from build123d import *

# Parameters (mm, degrees)
F0_W      = 111.801914
F0_H      = 111.801914
F1_DEPTH  = 57.15
F2_W      = 72.47591
F2_H      = 72.47591
F3_DEPTH  = 71.12
F4_W      = 21.19565
F4_H      = 21.19565
F5_DEPTH  = 76.2
F6_R      = 16.556677
F7_W      = 7.638184
F7_H      = 15.41857
F8_DEPTH  = 25.4
F8_FACE_W = 7.638184
F8_FACE_H = 15.41857
F9_DEPTH  = 27.432
F10_W     = 78.688562
F10_H     = 9.165822
F11_DEPTH = 8.89
F12_W     = 8.714252
F12_H     = 81.186646
F13_DEPTH = 8.636
F14_W     = 78.688562
F14_H     = 8.29689
F15_DEPTH = 15.748
F16_W     = 8.432022
F16_H     = 81.186646
F17_DEPTH = 12.446
F18_R     = 18.732784
F19_DEPTH = 1.778


with BuildPart() as f1:
    # F0 (on Top) → F1 (new body, symmetric)
    with BuildSketch(Plane.XY):
        Rectangle(F0_W, F0_H)
    extrude(amount=F1_DEPTH, both=True)

    # F2 (on face) → F3 (join)
    with BuildSketch(Plane.XZ.offset(55.900957)):
        Rectangle(F2_W, F2_H)
    extrude(amount=F3_DEPTH)

    # F4 (on face) → F5 (join)
    with BuildSketch(Plane.XZ.offset(127.020957)):
        Rectangle(F4_W, F4_H)
    extrude(amount=F5_DEPTH)

    # F6
    f6_edges = [f1.edges().sort_by_distance(p)[0] for p in [
        (-55.900957, 0, 57.15),
        (-55.900957, 0, -57.15),
        (55.900957, 0, -57.15),
        (55.900957, 0, 57.15),
        (36.237955, -127.020957, 0),
        (0, -127.020957, -36.237955),
        (-36.237955, -127.020957, 0),
        (0, -127.020957, 36.237955),
        (-36.237955, -91.460957, -36.237955),
        (36.237955, -91.460957, -36.237955),
        (36.237955, -91.460957, 36.237955),
        (-36.237955, -91.460957, 36.237955),
    ]]
    fillet(f6_edges, radius=F6_R)

    # F7 (on face) → F8 (join)
    with BuildSketch(Plane.XY.offset(57.15)):
        with Locations((-30.17084, 48.191672)):
            Rectangle(F7_W, F7_H)
    extrude(amount=F8_DEPTH)

    # F8_face (on face) → F9 (cut)
    with BuildSketch(Plane(origin=(-30.17084, 48.191672, 82.55), x_dir=(1, 0, 0), z_dir=(0, 0, 1))):
        Rectangle(F8_FACE_W, F8_FACE_H)
    extrude(amount=-F9_DEPTH, mode=Mode.SUBTRACT)

    # F10 (on face) → F11 (cut)
    with BuildSketch(Plane.XY.offset(57.15)):
        Rectangle(F10_W, F10_H)
    extrude(amount=-F11_DEPTH, mode=Mode.SUBTRACT)

    # F12 (on face) → F13 (cut)
    with BuildSketch(Plane(origin=(-55.900957, 0, 0), x_dir=(0, -1, 0), z_dir=(-1, 0, 0))):
        Rectangle(F12_W, F12_H)
    extrude(amount=-F13_DEPTH, mode=Mode.SUBTRACT)

    # F14 (on face) → F15 (cut)
    with BuildSketch(Plane(origin=(0, 0, -57.15), x_dir=(1, 0, 0), z_dir=(0, 0, -1))):
        Rectangle(F14_W, F14_H)
    extrude(amount=-F15_DEPTH, mode=Mode.SUBTRACT)

    # F16 (on face) → F17 (cut)
    with BuildSketch(Plane.YZ.offset(55.900957)):
        Rectangle(F16_W, F16_H)
    extrude(amount=-F17_DEPTH, mode=Mode.SUBTRACT)

    # F18 (on face) → F19 (join)
    with BuildSketch(Plane.XY.offset(36.237955)):
        with Locations((0, -89.04539)):
            Circle(F18_R)
    extrude(amount=F19_DEPTH)


solid = f1.part
CAD build for the part. Positions are in the model's coordinates, mm. A direction names the side the tool comes from. Give positions to 0.01 mm unless a question says otherwise; leave off trailing zeros. Order: outer loops, then holes, each group sorted by start corner. A loop starts at its lowest first (then second) coordinate and runs counter-clockwise, first axis right, second up. Notation, with made-up numbers: (75, 22) - (102, 22) arc R13 cw to (102, 37) - close; hole circle Ø6 at (-8.5, 50). An arc over 180 degrees is marked (long way). Answer in a Markdown table with one row per item.
1. Pull direction Y, two halves, no side cores. Call faces 1 (the flat face through (-1, 0, 48.26)), 2 (the flat face through (-47.265, 0, 1)), 3 (the flat face through (0, -203.221, 0)), 4 (the flat face through (-30, 48, 55.118)): pulls with the +Y half, pulls with the -Y half, needs draft (parallel to the pull), parting line crosses it, or undercut.
Data:
| item | result |
|---|---|
| face 1 | undercut |
| face 2 | undercut |
| face 3 | pulls with the -Y half |
| face 4 | needs draft |
2. Saw through at B-B, the plane y = 11.5. Give the cut face in (x, z).
Data:
| item | result |
|---|---|
| outline | (-55.9, -40.59) arc R16.56 ccw to (-39.34, -57.15) - (39.34, -57.15) arc R16.56 ccw to (55.9, -40.59) - (55.9, 40.59) arc R16.56 ccw to (39.34, 57.15) - (-39.34, 57.15) arc R16.56 ccw to (-55.9, 40.59) - close |
3. Flat gauge pins, fed straight in: pin 1 (2.5 mm diameter, centred on x = 51.5, y = 0, fed in from +Z); pin 2 (3 mm diameter, centred on x = -19, z = -10, fed in from -Y); pin 3 (10 mm diameter, centred on y = -116.5, z = 28.5, fed in from -X). Where does each tip first touch, or does it go through?
Data:
| item | result |
|---|---|
| pin 1 | stops at z = 53.05 |
| pin 2 | stops at y = -127.02 |
| pin 3 | stops at x = -35.23 |
4. Saw through at D-D, the plane x = 31.5. Give the cut face in (y, z).
Data:
| item | result |
|---|---|
| outline | (-122.06, -19.68) arc R11.59 ccw to (-110.46, -31.28) - (-55.9, -31.28) - (-55.9, -57.15) - (-4.15, -57.15) - (-4.15, -41.4) - (4.15, -41.4) - (4.15, -57.15) - (55.9, -57.15) - (55.9, 57.15) - (4.58, 57.15) - (4.58, 48.26) - (-4.58, 48.26) - (-4.58, 57.15) - (-55.9, 57.15) - (-55.9, 31.28) - (-110.46, 31.28) arc R11.59 ccw to (-122.06, 19.68) - close |
5. Probe probe 1 along Y at (x, z) = (47, -26.5); probe 2 along Y at (x, z) = (-9.5, 50); probe 3 along X at (y, z) = (-72, 16). List the from-to ranges inside material, lowest first. Write a range as [from, to].
Data:
| item | result |
|---|---|
| probe 1 | y = [-55.9, -4.22], [4.22, 55.9] |
| probe 2 | y = [-55.9, -4.58], [4.58, 55.9] |
| probe 3 | x = [-36.24, 36.24] |
6. Tool access for faces 5 (the flat face through (-1, 0, -41.402)), 6 (the flat face through (-52, 0, 40.593)), 7 (the cylindrical face through (-31.259, -83.565, -31.517)), 8 (the flat face through (50, 0, 40.593)): list every direction of +Z, -Z, +X, -X, +Y, -Y with a clear straight run to the whole face (end or side of a thin tool).
Data:
| item | result |
|---|---|
| face 5 | -Z |
| face 6 | -X |
| face 7 | -Z, -X, -Y |
| face 8 | +X |
7. Saw through at C-C, the plane x = 0. Give the cut face in (y, z), plus the area to 3 significant figures.
Data:
| item | result |
|---|---|
| outline | (-203.22, -10.6) - (-127.02, -10.6) - (-127.02, -19.68) arc R16.56 ccw to (-110.46, -36.24) - (-55.9, -36.24) - (-55.9, -57.15) - (-4.15, -57.15) - (-4.15, -41.4) - (4.15, -41.4) - (4.15, -57.15) - (55.9, -57.15) - (55.9, 57.15) - (4.58, 57.15) - (4.58, 48.26) - (-4.58, 48.26) - (-4.58, 57.15) - (-55.9, 57.15) - (-55.9, 36.24) - (-70.31, 36.24) - (-70.31, 38.02) - (-107.78, 38.02) - (-107.78, 36.24) - (-110.46, 36.24) arc R16.56 ccw to (-127.02, 19.68) - (-127.02, 10.6) - (-203.22, 10.6) - close |
| area | 19,300 mm² |
8. Saw through at A-A, the plane z = 1. Give the cut face in (x, y), plus the area to 3 significant figures.
Data:
| item | result |
|---|---|
| outline | (-55.9, -55.9) - (-36.24, -55.9) - (-36.24, -110.46) arc R16.56 ccw to (-19.68, -127.02) - (-10.6, -127.02) - (-10.6, -203.22) - (10.6, -203.22) - (10.6, -127.02) - (19.68, -127.02) arc R16.56 ccw to (36.24, -110.46) - (36.24, -55.9) - (55.9, -55.9) - (55.9, -4.22) - (43.45, -4.22) - (43.45, 4.22) - (55.9, 4.22) - (55.9, 55.9) - (-55.9, 55.9) - (-55.9, 4.36) - (-47.26, 4.36) - (-47.26, -4.36) - (-55.9, -4.36) - close |
| area | 19,000 mm² |
